from build123d import *

# Parameters (mm, degrees)
BOSS_EXTRUDE1_DEPTH = 322.5
FILLET1_R           = 1


with BuildPart() as part:
    # Sketch2 → Boss-Extrude1 (new body)
    with BuildSketch(Plane(origin=(0, 0, 0), x_dir=(0, 0, -1), z_dir=(1, 0, 0))):
        with BuildLine():
            Line((2.5, 5.837165408), (2.5, 4.35))
            Line((2.5, 4.35), (-2.5, 4.35))
            Line((-2.5, 4.35), (-2.5, 5.837165408))
            ThreePointArc((-2.5, 5.837165408), (0, -6.35), (2.5, 5.837165408))
        make_face()
    extrude(amount=BOSS_EXTRUDE1_DEPTH)

    # Fillet1
    fillet1_edges = [part.edges().sort_by_distance(p)[0] for p in [
        (0, -6.35, 0),
        (322.5, -6.35, 0),
    ]]
    fillet(fillet1_edges, radius=FILLET1_R)


solid = part.part
Read the model definition and answer for the solid it produces. Units are mm, in the model's axes. Round coordinates to 2 decimals unless told otherwise and drop trailing zeros. Order: outer loops, then holes, each group sorted by start corner. A loop starts at its lowest first (then second) coordinate and runs counter-clockwise, first axis right, second up.
1) Straight lines are drawn through the part: L1, parallel to Y at x = 169, z = -3.5; L2, parallel to X at y = 3, z = 4.5; L3, parallel to Z at x = 113.5, y = 5.5. For each, find the intervals that lie inside material, in ascending order.
2) The part is cut by section B-B on x = 142.5. Write down the section's boundary in (y, z), plus the area to 3 significant figures.
3) Flat-ended cylindrical pins translate along their axes: pin 1 (1.6 mm diameter, centred on x = 115, y = 5, fed in from -Z); pin 2 (1 mm diameter, centred on x = 82, y = -1.5, fed in from -Z); pin 3 (1.5 mm diameter, centred on x = 159.5, z = -1.5, fed in from -Y). Find the tip coordinate at first contact, or state that the pin passes through.
4) The part is cut by section A-A on z = 0. Write down the section's boundary in (x, y).
5) The mould has two halves that part along Z. Classify faces 1 (the face through (159, 4.35, 0)), 2 (the face through (0, 0, 0)), 3 (the face through (159.006, -6.345, 0.243)): released by +Z, released by -Z, zero draft, split by the parting line, or undercut.
Resolved:
1. L1: y = -5.3 to 5.3
1. L2: x = 0 to 322.5
1. L3: z = -3.17 to -2.5, 2.5 to 3.17
2. outline: (4.35, -2.5) - (4.35, 2.5) - (5.84, 2.5) arc R6.35 ccw (long way) to (5.84, -2.5) - close
2. area: 118 mm2
3. pin 1: stops at z = -4.76
3. pin 2: stops at z = -6.27
3. pin 3: stops at y = -6.31
4. outline: (0, -5.35) arc R1 ccw to (1, -6.35) - (321.5, -6.35) arc R1 ccw to (322.5, -5.35) - (322.5, 4.35) - (0, 4.35) - close
5. face 1: undercut
5. face 2: zero draft
5. face 3: split by the parting line
